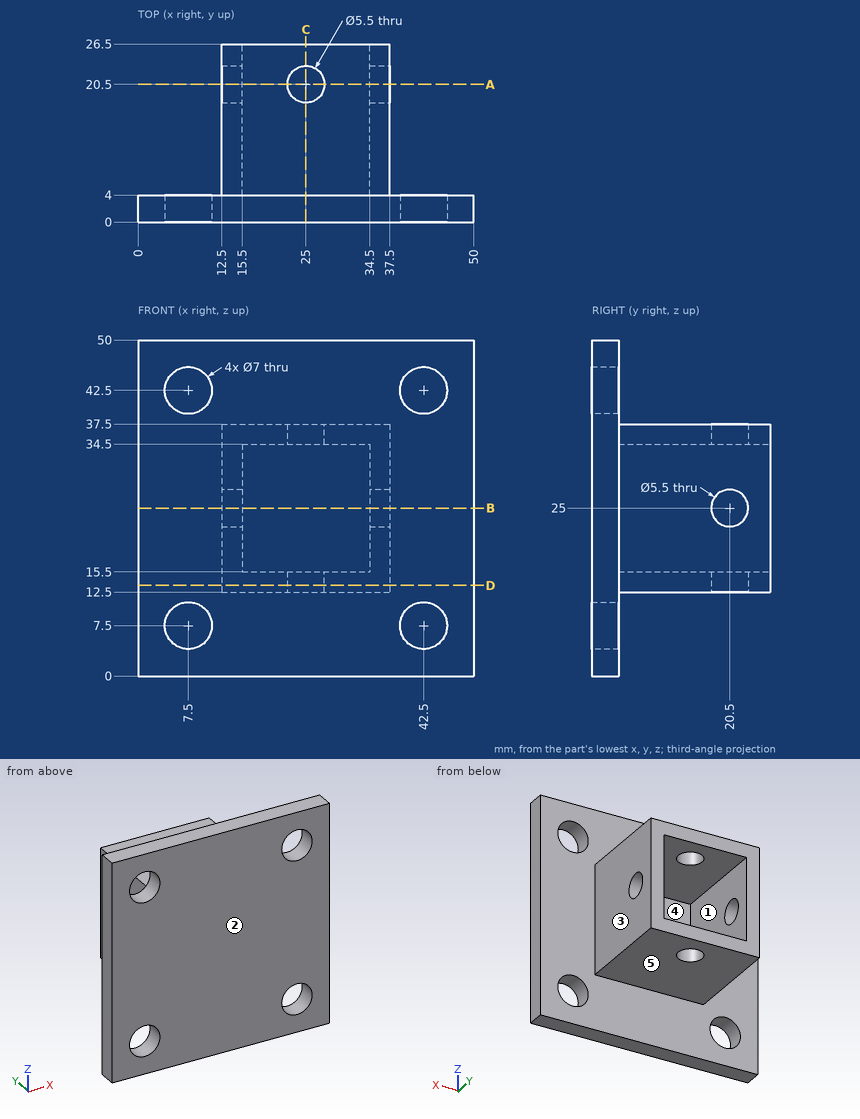
Could you check a few things on this drawing? It's one solid part, dimensions in mm from its lowest x, y, z. A direction names the side the tool comes from. Round coordinates to 2 decimals unless told otherwise and drop trailing zeros. Write each loop counter-clockwise with the first axis right and the second up, starting at its lowest first coordinate (ties: lowest second). Pieces come first, ordered by that corner, then holes.
Q1. If we section it at A-A on y = 20.5: Write out the boundary of the cut face in (x, z).
Q2. Please list where these lines run through material, in increasing order: probe 1 along X at (y, z) = (3.15, 42.5); probe 2 along Z at (x, y) = (19.5, 15).
Q3. If we section it at B-B on z = 25: Write out the boundary of the cut face in (x, y).
Q4. Will these pins go through, and if not, where does the flat tip stop? P1, Ø5.5, axis at y = 19.5, z = 25, coming from the -X side; P2, Ø6, axis at x = 42.5, y = 9, coming from the -Z side; P3, Ø10, axis at x = 31, z = 23.5, coming from the +Y side; P4, Ø1, axis at y = 12, z = 27, coming from the +X side.
Q5. If we section it at C-C on x = 25: Write out the boundary of the cut face in (y, z).
Q6. Which directions (+Z, -Z, +X, -X, +Y, -Y) give clear straight access to the entire face, cutting with the end or side of a thin tool? Please do the marked faces 1 and 2.
Q7. If we mould it in two halves opening along Z, with no side actions, what happens to the marked faces 3, 4 and 5? For each: +Z half, -Z half, draft (parallel to the pull), parting line (faces both ways), or undercut.
Q8. If we section it at D-D on z = 13.5: Write out the boundary of the cut face in (x, y).
Answer below:
1. outline: (12.5, 12.5) - (22.25, 12.5) - (22.25, 15.5) - (15.5, 15.5) - (15.5, 22.25) - (12.5, 22.25) - close; (12.5, 27.75) - (15.5, 27.75) - (15.5, 34.5) - (22.25, 34.5) - (22.25, 37.5) - (12.5, 37.5) - close; (27.75, 12.5) - (37.5, 12.5) - (37.5, 22.25) - (34.5, 22.25) - (34.5, 15.5) - (27.75, 15.5) - close; (27.75, 34.5) - (34.5, 34.5) - (34.5, 27.75) - (37.5, 27.75) - (37.5, 37.5) - (27.75, 37.5) - close
2. probe 1: x = 0 to 4, 11 to 39, 46 to 50
2. probe 2: z = 12.5 to 15.5, 34.5 to 37.5
3. outline: (0, 0) - (50, 0) - (50, 4) - (37.5, 4) - (37.5, 17.75) - (34.5, 17.75) - (34.5, 4) - (15.5, 4) - (15.5, 17.75) - (12.5, 17.75) - (12.5, 4) - (0, 4) - close; (12.5, 23.25) - (15.5, 23.25) - (15.5, 26.5) - (12.5, 26.5) - close; (34.5, 23.25) - (37.5, 23.25) - (37.5, 26.5) - (34.5, 26.5) - close
4. P1: stops at x = 12.5
4. P2: passes through
4. P3: stops at y = 26.5
4. P4: stops at x = 37.5
5. outline: (0, 0) - (4, 0) - (4, 12.5) - (17.75, 12.5) - (17.75, 15.5) - (4, 15.5) - (4, 34.5) - (17.75, 34.5) - (17.75, 37.5) - (4, 37.5) - (4, 50) - (0, 50) - close; (23.25, 12.5) - (26.5, 12.5) - (26.5, 15.5) - (23.25, 15.5) - close; (23.25, 34.5) - (26.5, 34.5) - (26.5, 37.5) - (23.25, 37.5) - close
6. face 1: +Y
6. face 2: +Z, -Z, +X, -X, -Y
7. face 3: draft
7. face 4: undercut
7. face 5: -Z half
8. outline: (0, 0) - (50, 0) - (50, 4) - (37.5, 4) - (37.5, 26.5) - (12.5, 26.5) - (12.5, 4) - (0, 4) - close; hole circle Ø5.5 at (25, 20.5)
